Check sheet for the modelled part. Datum: model origin and axes. Units: mm. A direction names the side the tool comes from. Round coordinates to 2 decimals unless told otherwise and drop trailing zeros. Order: outer loops, then holes, each group sorted by start corner. A loop starts at its lowest first (then second) coordinate and runs counter-clockwise, first axis right, second up. Notation, with made-up numbers: (-32.5, 37) -> (-11.5, 37) arc R33 cw to (-11.5, 76) -> close; hole circle Ø8 at (26, 14). An arc over 180 degrees is marked (long way). Answer as CSV lines item,"result". Start each with the question number.
from build123d import *

# Parameters (mm, degrees)
F0_W     = 1.4192797244
F0_H     = 0.7559135556
F0_W_2   = 1.5276372433
F0_H_2   = 0.821922149
F1_DEPTH = 5.08
F3_D     = 5.08
F16_D    = 2.54
F17_D    = 2.54
F18_D    = 2.54
F19_D    = 2.54
F20_D    = 2.54
F21_D    = 2.54
F22_D    = 2.54
F23_D    = 2.54
F24_D    = 2.54
F25_D    = 2.54
F26_D    = 2.54
F27_D    = 2.54


with BuildPart() as f1:
    # F0 (on Front) → F1 (new body)
    with BuildSketch(Plane.XZ):
        Polygon((-22.9968726635, 42.3126220703), (-24.0396112204, 42.3126220703), (-23.9130631089, 37.6422533683), (-27.5855498346, 40.0842883347), (-29.8122577369, 36.7356240749), (-23.9130631089, 32.8129306436), (-23.9130631089, 30.5526573211), (-23.9130631089, 25.2665821463), (-28.3773863184, 27.9790678606), (-30.1533350523, 29.0581195654), (-30.897045508, 36.2559482455), (-34.5488109312, 35.8786322176), (-34.5488109312, 31.4557254833), (-38.2708328584, 33.4987355549), (-38.8486688201, 32.4460152822), (-39.5886734839, 31.0978508149), (-40.0970317423, 30.1717072725), (-36.5123793412, 28.2040990472), (-40.4995033926, 25.8957650515), (-38.450665772, 22.3568622023), (-32.2511233389, 25.4756510258), (-30.4993555618, 24.4352070583), (-25.9755142033, 21.7483192682), (-30.4993555618, 19.148359909), (-32.3296703771, 18.0964343976), (-38.2196328624, 21.207898243), (-40.0970317423, 17.6540054381), (-36.1978308162, 15.5941921986), (-40.1960664707, 13.2942146556), (-39.6006508042, 12.2591557897), (-38.790906044, 10.8515114494), (-38.2163748145, 9.8527576774), (-34.3487829088, 12.0775826495), (-34.5557542526, 7.6535682905), (-30.6067895144, 7.4688214809), (-30.2744992077, 14.5715298131), (-28.5829074003, 15.5766311017), (-23.9130631089, 18.3513350785), (-23.9130631089, 12.9318498075), (-23.9130631089, 10.946790142), (-29.8032763032, 6.8207080641), (-27.4943839759, 3.5246349871), (-23.9130631089, 6.0333427973), (-23.9130631089, 1.2797450181), (-22.7054376155, 1.2797450181), (-21.1778003722, 1.2797450181), (-19.952988252, 1.2797450181), (-19.952988252, 6.044047419), (-16.3245014846, 3.5494628828), (-14.3590718508, 6.9133723155), (-20.0663805008, 10.9954206273), (-20.0550059627, 13.2019692024), (-20.0285818428, 18.3279886842), (-15.7154238075, 15.6576944664), (-13.8587799241, 14.5082384562), (-13.3001293296, 7.4345099906), (-9.3699013814, 7.7449013479), (-9.7278654156, 12.2775025894), (-5.8548050001, 10.0505026057), (-5.4199136441, 10.8068387119), (-4.568640864, 12.2873195971), (-3.9422987452, 13.3766150102), (-7.6739792712, 15.7493855804), (-3.9422987452, 17.6644706865), (-5.6661837734, 21.2469194084), (-12.0242014527, 18.1874223053), (-13.6816729537, 19.189614399), (-18.1910004467, 21.9161845744), (-13.6816729537, 24.5599445899), (-11.6887243355, 25.7283844245), (-5.7599901473, 22.6144351328), (-3.9422987452, 26.0751880705), (-7.6739792712, 28.0351787806), (-3.9422987452, 30.5491588676), (-4.5895827798, 31.7159527215), (-5.3169873732, 33.0271718518), (-5.809597671, 33.9151509106), (-9.8331745535, 31.6830538959), (-9.5743191002, 36.0260785228), (-13.4583404288, 36.2575761974), (-13.8885816559, 29.0390755981), (-15.4547147461, 28.084917372), (-20.0873508675, 25.2625085413), (-20.0873508675, 30.6201688945), (-20.0873508675, 32.5695575383), (-14.4622381777, 36.7356240749), (-16.7762544006, 39.8600585759), (-20.3607678413, 37.7848148346), (-20.3607678413, 42.3126220703), (-21.5775929391, 42.3126220703), align=None)
        with Locations((-22.2872328013, 42.6905788481)):
            Rectangle(F0_W, F0_H)
        Polygon((-23.9130631089, 30.5526573211), (-23.9130631089, 32.8129306436), (-30.1533350523, 29.0581195654), (-28.3773863184, 27.9790678606), align=None)
        Polygon((-13.8885816559, 29.0390755981), (-20.0873508675, 32.5695575383), (-20.0873508675, 30.6201688945), (-15.4547147461, 28.084917372), align=None)
        Polygon((-39.5886734839, 31.0978508149), (-38.8486688201, 32.4460152822), (-39.664609785, 32.8938835758), (-40.4046144488, 31.5457191085), align=None)
        Polygon((-4.5909064128, 33.4299684657), (-5.3169873732, 33.0271718518), (-4.5895827798, 31.7159527215), (-3.8635018193, 32.1187493355), align=None)
        Polygon((-30.4993555618, 24.4352070583), (-32.2511233389, 25.4756510258), (-32.3296703771, 18.0964343976), (-30.4993555618, 19.148359909), align=None)
        Polygon((-12.0242014527, 18.1874223053), (-11.6887243355, 25.7283844245), (-13.6816729537, 24.5599445899), (-13.6816729537, 19.189614399), align=None)
        Polygon((-38.790906044, 10.8515114494), (-39.6006508042, 12.2591557897), (-40.3208764938, 11.8448473159), (-39.5111317337, 10.4372029756), align=None)
        Polygon((-3.5707916424, 11.713558808), (-4.568640864, 12.2873195971), (-5.4199136441, 10.8068387119), (-4.4220644224, 10.2330779228), align=None)
        Polygon((-28.5829074003, 15.5766311017), (-30.2744992077, 14.5715298131), (-23.9130631089, 10.946790142), (-23.9130631089, 12.9318498075), align=None)
        Polygon((-20.0663805008, 10.9954206273), (-13.8587799241, 14.5082384562), (-15.7154238075, 15.6576944664), (-20.0550059627, 13.2019692024), align=None)
        with Locations((-21.9416189939, 0.8687839436)):
            Rectangle(F0_W_2, F0_H_2)
    extrude(amount=F1_DEPTH)

    # F3 (through all)
    with Locations(Plane(origin=(0, 0, 0), x_dir=(1, 0, 0), z_dir=(0, 1, 0))):
        with Locations((-22.2109630704, -21.9656527042)):
            Hole(F3_D / 2)

    # F16 (through all)
    with Locations(Plane(origin=(0, 0, 0), x_dir=(1, 0, 0), z_dir=(0, 1, 0))):
        with Locations((-22.1980046481, -30.305903405)):
            Hole(F16_D / 2)

    # F17 (through all)
    with Locations(Plane(origin=(0, 0, 0), x_dir=(1, 0, 0), z_dir=(0, 1, 0))):
        with Locations((-22.0177676529, -26.8813967705)):
            Hole(F17_D / 2)

    # F18 (through all)
    with Locations(Plane(origin=(0, 0, 0), x_dir=(1, 0, 0), z_dir=(0, 1, 0))):
        with Locations((-18.0525481701, -24.2679584771)):
            Hole(F18_D / 2)

    # F19 (through all)
    with Locations(Plane(origin=(0, 0, 0), x_dir=(1, 0, 0), z_dir=(0, 1, 0))):
        with Locations((-15.3489904478, -25.9802117944)):
            Hole(F19_D / 2)

    # F20 (through all)
    with Locations(Plane(origin=(0, 0, 0), x_dir=(1, 0, 0), z_dir=(0, 1, 0))):
        with Locations((-18.2327851653, -20.0323835015)):
            Hole(F20_D / 2)

    # F21 (through all)
    with Locations(Plane(origin=(0, 0, 0), x_dir=(1, 0, 0), z_dir=(0, 1, 0))):
        with Locations((-15.529227443, -18.0497746915)):
            Hole(F21_D / 2)

    # F22 (through all)
    with Locations(Plane(origin=(0, 0, 0), x_dir=(1, 0, 0), z_dir=(0, 1, 0))):
        with Locations((-22.0177676529, -17.4189452082)):
            Hole(F22_D / 2)

    # F23 (through all)
    with Locations(Plane(origin=(0, 0, 0), x_dir=(1, 0, 0), z_dir=(0, 1, 0))):
        with Locations((-22.2881231457, -13.633963652)):
            Hole(F23_D / 2)

    # F24 (through all)
    with Locations(Plane(origin=(0, 0, 0), x_dir=(1, 0, 0), z_dir=(0, 1, 0))):
        with Locations((-26.3434592634, -19.3114355206)):
            Hole(F24_D / 2)

    # F25 (through all)
    with Locations(Plane(origin=(0, 0, 0), x_dir=(1, 0, 0), z_dir=(0, 1, 0))):
        with Locations((-29.1371364146, -17.5090637058)):
            Hole(F25_D / 2)

    # F26 (through all)
    with Locations(Plane(origin=(0, 0, 0), x_dir=(1, 0, 0), z_dir=(0, 1, 0))):
        with Locations((-26.5236981213, -24.4481954724)):
            Hole(F26_D / 2)

    # F27 (through all)
    with Locations(Plane(origin=(0, 0, 0), x_dir=(1, 0, 0), z_dir=(0, 1, 0))):
        with Locations((-29.4976104051, -26.3406857848)):
            Hole(F27_D / 2)


solid = f1.part
1) Section check C-C on x = -27. Count the separate pieces of the cut face and the enclosed holes in it, then the cut area to 3 significant figures.
2) Mould release check, pull along Z, two halves, no side actions. Record for faces 6 (the face through (-32.609, -2.504, 7.562)), 7 (the face through (-32.7, -2.5, 36.07)), 8 (the face through (-39.145, -2.504, 19.456)): released by +Z, released by -Z, zero draft, split by the parting line, or undercut.
3) Access from +Z, -Z, +X, -X, +Y, -Y to the whole of each face (thin tool, end or side, straight path). Record for faces 1 (the face through (-39.92, -2.5, 11.15)), 2 (the face through (-21, -3, 1.28)), 3 (the face through (-4.928, -2.504, 10.524)), 4 (the face through (-16.945, -2.504, 30.78)), 5 (the face through (-21, -3, 42.313)).
4) Depth check by flat-ended pin: pin 1 Ø0.6 at (y, z) = (-3.5, 42.5) entering from +X; pin 2 Ø2 at (y, z) = (-4, 35.5) entering from +X; pin 3 Ø0.7 at (y, z) = (-2, 0.5) entering from +X; pin 4 Ø3 at (x, y) = (-21, -0.5) entering from -Z. Enter the tip coordinate at first touch or a pass-through.
5) Material ranges on line 1 along X through (y, z) = (-1.35, 31); line 2 along Z through (x, y) = (-6, -1.9) (1 decimal); line 3 along X through (y, z) = (-3.15, 9), recorded low to high.
6) Section check A-A on z = 5.5. Record the cut outline in (x, y), then the cut area to 3 significant figures.
7) Section check B-B on x = -7. Record the cut outline in (y, z), then the cut area to 3 significant figures.
Solutions:
1,separate pieces,"8"
1,enclosed holes,"0"
1,area,"95.5 mm^2"
2,face 6,"released by -Z"
2,face 7,"released by +Z"
2,face 8,"undercut"
3,face 1,"-Z, -X, +Y, -Y"
3,face 2,"-Z, +X, +Y, -Y"
3,face 3,"-Z, +Y, -Y"
3,face 4,"+Y, -Y"
3,face 5,"+Z, +X, +Y, -Y"
4,pin 1,"stops at x = -20.36"
4,pin 2,"stops at x = -9.57"
4,pin 3,"stops at x = -21.18"
4,pin 4,"stops at z = 0.46"
5,line 1,"x = -39.64 to -30.35, -26.93 to -23.26, -21.13 to -17.33, -13.77 to -4.19"
5,line 2,"z = 10.1 to 14.7, 16.6 to 21.1, 22.7 to 27.2, 29.2 to 33.8"
5,line 3,"x = -34.49 to -30.54, -26.69 to -17.28, -13.42 to -9.47"
6,outline,"(-28.88, -5.08) -> (-24.67, -5.08) -> (-24.67, 0) -> (-28.88, 0) -> close; (-23.91, -5.08) -> (-19.95, -5.08) -> (-19.95, 0) -> (-23.91, 0) -> close; (-19.16, -5.08) -> (-15.18, -5.08) -> (-15.18, 0) -> (-19.16, 0) -> close"
6,area,"61.7 mm^2"
7,outline,"(-5.08, 10.71) -> (0, 10.71) -> (0, 15.32) -> (-5.08, 15.32) -> close; (-5.08, 16.1) -> (0, 16.1) -> (0, 20.61) -> (-5.08, 20.61) -> close; (-5.08, 23.27) -> (0, 23.27) -> (0, 27.68) -> (-5.08, 27.68) -> close; (-5.08, 28.49) -> (0, 28.49) -> (0, 33.25) -> (-5.08, 33.25) -> close"
7,area,"93.0 mm^2"
